The listing builds one solid part. Answer for the finished solid, in the listing's coordinates (mm). Face numbers are marked on the shaded views. A direction names the side the tool comes from. Give positions to 0.01 mm unless a question says otherwise; leave off trailing zeros. Order: outer loops, then holes, each group sorted by start corner. A loop starts at its lowest first (then second) coordinate and runs counter-clockwise, first axis right, second up. Notation, with made-up numbers: (46.25, 26) -> (82.25, 26) arc R21 ccw to (82.25, 46) -> close; hole circle Ø5 at (44, -34.75). An arc over 180 degrees is marked (long way). Write item = value, one per line. Start each with the question number.
```python
from build123d import *

# Parameters (mm, degrees)
SKETCH1_R           = 11
SKETCH1_R_2         = 5.1
BOSS_EXTRUDE1_DEPTH = 10
SKETCH2_R           = 1.75
CUT_EXTRUDE1_DEPTH  = 19.493242009
BOSS_EXTRUDE2_START = 11
SKETCH3_W           = 22
SKETCH3_H           = 10
BOSS_EXTRUDE2_DEPTH = 10.16
BOSS_EXTRUDE3_REACH = 28.552
SKETCH5_W           = 22
SKETCH5_H           = 10
SKETCH6_W           = 10.16
SKETCH6_H           = 10.16
CUT_EXTRUDE2_DEPTH  = 26.860116009
SKETCH7_R           = 1.75
CUT_EXTRUDE3_DEPTH  = 33.120797001


with BuildPart() as part:
    # Sketch1 → Boss-Extrude1 (new body)
    with BuildSketch(Plane.XY):
        Circle(SKETCH1_R)
        Circle(SKETCH1_R_2, mode=Mode.SUBTRACT)
    extrude(amount=BOSS_EXTRUDE1_DEPTH)

    # Sketch2 → Cut-Extrude1 (cut, through all)
    with BuildSketch(Plane.XY.offset(10)):
        with Locations((0, 8)):
            Circle(SKETCH2_R)
        with Locations((8, 0)):
            Circle(SKETCH2_R)
        with Locations((0, -8)):
            Circle(SKETCH2_R)
        with Locations((-8, 0)):
            Circle(SKETCH2_R)
    extrude(amount=-CUT_EXTRUDE1_DEPTH, mode=Mode.SUBTRACT)

    # Sketch5 → Boss-Extrude3 (add, up to next)
    with BuildSketch(Plane.XZ.offset(-11), mode=Mode.PRIVATE) as boss_extrude3_sk1:
        with Locations((0, 5)):
            Rectangle(SKETCH5_W, SKETCH5_H)
    boss_extrude3_tool1 = extrude(boss_extrude3_sk1.sketch, amount=BOSS_EXTRUDE3_REACH, mode=Mode.PRIVATE) - part.part


with BuildPart() as body_2:
    # Sketch3 → Boss-Extrude2 (new body)
    with BuildSketch(Plane(origin=(0, 0, 0), x_dir=(1, 0, 0), z_dir=(0, 1, 0)).offset(BOSS_EXTRUDE2_START)):
        with Locations((0, -5)):
            Rectangle(SKETCH3_W, SKETCH3_H)
    extrude(amount=BOSS_EXTRUDE2_DEPTH)


with BuildPart() as part_1:
    add(part.part)

    add(body_2.part)  # Boss-Extrude3 merges body 2
    add(boss_extrude3_tool1.solids().sort_by_distance((0, 11, 5))[0])
    add(boss_extrude3_tool1.solids().sort_by_distance((0, 11, 5))[1])

    # Sketch6 → Cut-Extrude2 (cut, through all)
    with BuildSketch(Plane.XY.offset(10)):
        with Locations((0, 16.08)):
            Rectangle(SKETCH6_W, SKETCH6_H)
    extrude(amount=-CUT_EXTRUDE2_DEPTH, mode=Mode.SUBTRACT)

    # Sketch7 → Cut-Extrude3 (cut, through all)
    with BuildSketch(Plane(origin=(11, 0, 0), x_dir=(0, 0, -1), z_dir=(1, 0, 0))):
        with Locations((-5, 16.08)):
            Circle(SKETCH7_R)
    extrude(amount=-CUT_EXTRUDE3_DEPTH, mode=Mode.SUBTRACT)


solid = part_1.part
```
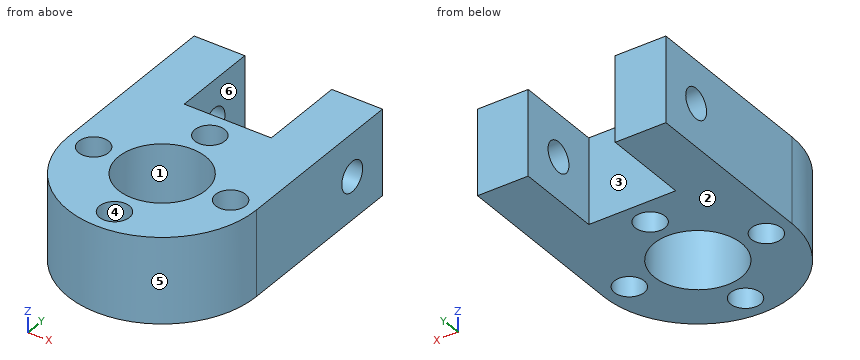
Item 1: Consider L1, parallel to Y at x = 0, z = 4.5; L2, parallel to X at y = 17.5, z = 7; L3, parallel to Y at x = -6.6, z = 5. Determine where each line is inside the solid, lowest interval first. Write a range as from..to.
Item 2: Flat-ended cylindrical pins translate along their axes: pin 1 (2 mm diameter, centred on y = 16.08, z = 5, fed in from +X); pin 2 (2 mm diameter, centred on x = -7, z = 3.5, fed in from -Y). Find the tip coordinate at first contact, or state that the pin passes through.
Item 3: A cutting plane is placed at D-D, the plane x = -6.75. Write down the section's boundary in (y, z).
Item 4: A cutting plane is placed at B-B, the plane y = 8. Write down the section's boundary in (x, z), plus the area to 3 significant figures.
Item 5: Which of the six approach directions +Z, -Z, +X, -X, +Y, -Y give full straight-line access (tool end or side, diameter ignored) to the marked faces 5 and 6?
Item 6: A cutting plane is placed at A-A, the plane z = 5. Write down the section's boundary in (x, y).
Item 7: The mould has two halves that part along Y. Classify the marked faces 1, 2, 3 and 4: +Y half, -Y half, draft (parallel to the pull), parting line (faces both ways), or undercut.
Item 8: A cutting plane is placed at C-C, the plane x = 0. Write down the section's boundary in (y, z).
Check values:
q1.L1 = -11..-9.75, -6.25..-5.1, 5.1..6.25, 9.75..11
q1.L2 = -11..-5.08, 5.08..11
q1.L3 = -8.8..-1.05, 1.05..14.33, 17.83..21.16
q2.pin_1 = through
q2.pin_2 = -9.22
q3.outline = (-8.69, 0) -> (-1.22, 0) -> (-1.22, 10) -> (-8.69, 10) -> close; (1.22, 0) -> (21.16, 0) -> (21.16, 10) -> (1.22, 10) -> close; hole circle Ø3.5 at (16.08, 5)
q4.outline = (-11, 0) -> (-1.75, 0) -> (-1.75, 10) -> (-11, 10) -> close; (1.75, 0) -> (11, 0) -> (11, 10) -> (1.75, 10) -> close
q4.area = 185 mm^2
q5.face_5 = +Z, -Z, -Y
q5.face_6 = +Z, -Z, +Y
q6.outline = (-11, 0) arc R11 ccw to (11, 0) -> (11, 14.33) -> (5.08, 14.33) -> (5.08, 11) -> (-5.08, 11) -> (-5.08, 14.33) -> (-11, 14.33) -> close; (-11, 17.83) -> (-5.08, 17.83) -> (-5.08, 21.16) -> (-11, 21.16) -> close; (5.08, 17.83) -> (11, 17.83) -> (11, 21.16) -> (5.08, 21.16) -> close; hole circle Ø3.5 at (-8, 0); hole circle Ø10.2 at (0, 0); hole circle Ø3.5 at (0, -8); hole circle Ø3.5 at (0, 8); hole circle Ø3.5 at (8, 0)
q7.face_1 = undercut
q7.face_2 = draft
q7.face_3 = +Y half
q7.face_4 = undercut
q8.outline = (-11, 0) -> (-9.75, 0) -> (-9.75, 10) -> (-11, 10) -> close; (-6.25, 0) -> (-5.1, 0) -> (-5.1, 10) -> (-6.25, 10) -> close; (5.1, 0) -> (6.25, 0) -> (6.25, 10) -> (5.1, 10) -> close; (9.75, 0) -> (11, 0) -> (11, 10) -> (9.75, 10) -> close
